The model under review builds one solid part; all positions refer to its coordinate system, in mm. Give positions to 0.01 mm unless a question says otherwise; leave off trailing zeros. Loops run counter-clockwise (first coordinate to the right, second up) from the corner with the lowest first, then second, coordinate; pieces in that order, holes last. Notation, with made-up numbers: (16, 27) - (20, 27) arc R23 ccw to (20, 59) - close; hole circle Ø9 at (53.5, 85). An arc over 180 degrees is marked (long way). Return JSON: item names as keys, results as strings. Group by question number.
```python
from build123d import *

# Parameters (mm, degrees)
SKETCH1_W                                 = 63.5
SKETCH1_H                                 = 19.05
BOSS_EXTRUDE1_DEPTH                       = 1.27
CSK_FOR_4_FLAT_HEAD_MACHINE_SCREW_2_COUNT = 2
CSK_FOR_4_FLAT_HEAD_MACHINE_SCREW_2_PITCH = 51.93240976
FILLET2_R                                 = 0.254


with BuildPart() as part:
    # Sketch1 → Boss-Extrude1 (new body)
    with BuildSketch(Plane(origin=(0, 0, 0), x_dir=(1, 0, 0), z_dir=(0, 1, 0))):
        with Locations((0, 21.324911643)):
            Rectangle(SKETCH1_W, SKETCH1_H)
    extrude(amount=BOSS_EXTRUDE1_DEPTH)

    # Sketch15 → CSK for #4 Flat Head Machine Screw (100)2 (revolve, cut)
    with BuildSketch(Plane(origin=(-25.96620488, 1.27, -21.930009473), x_dir=(0, 0, 1), z_dir=(1, 0, 0))):
        Polygon((0, 0), (0, 1.27), (1.63195, 1.27), (1.63195, 1.028358553), (2.8575, 0), align=None)
    csk_for_4_flat_head_machine_screw_100 = revolve(axis=Axis((-25.96620488, 7.62, -21.930009473), (0, -1, 0)), mode=Mode.SUBTRACT)

    # CSK for _4 Flat Head Machine Screw _ 2: CSK for #4 Flat Head Machine Screw (100)2 ×2
    with Locations(*[(i * CSK_FOR_4_FLAT_HEAD_MACHINE_SCREW_2_PITCH, 0, 0) for i in range(1, CSK_FOR_4_FLAT_HEAD_MACHINE_SCREW_2_COUNT)]):
        add(csk_for_4_flat_head_machine_screw_100, mode=Mode.SUBTRACT)

    # Fillet2
    fillet2_edges = [part.edges().sort_by_distance(p)[0] for p in [
        (-31.75, 1.27, -21.324911643),
        (0, 1.27, -11.799911643),
        (31.75, 1.27, -21.324911643),
        (0, 1.27, -30.849911643),
    ]]
    fillet(fillet2_edges, radius=FILLET2_R)


solid = part.part
```
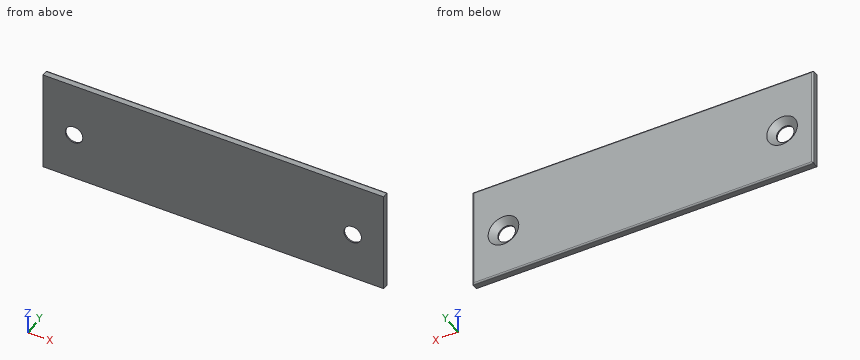
1) To check wall thickness, follow line 1 (X direction, y = 1.05, z = -19.75); line 2 (Z direction, x = -26, y = 0.1); line 3 (Z direction, x = -24, y = 0.85). State the ranges of each line that lie inside material, in increasing order.
2) For pin 1 Ø2 at (x, z) = (25.97, -21.93) entering from -Y; pin 2 Ø5 at (x, z) = (-25.97, -21.93) entering from +Y, all flat-tipped, find the tip position at first contact; note any pin that passes through.
3) We need section B-B, the plane z = -22.75. Count the separate pieces of the cut face and the enclosed holes in it, plus the area to 3 significant figures.
4) We need section A-A, the plane y = 0.75. Write out the cut boundary in (x, z), plus the area to 3 significant figures.
Findings:
{
 "1": {"line 1": "x = -31.75 to -27.37, -24.56 to 24.56, 27.37 to 31.75", "line 2": "z = -30.85 to -23.56, -20.3 to -11.8", "line 3": "z = -30.85 to -23.23, -20.63 to -11.8"},
 "2": {"pin 1": "passes through", "pin 2": "stops at y = 0.97"},
 "3": {"separate pieces": "3", "enclosed holes": "0", "area": "70.7 mm^2"},
 "4": {"outline": "(-31.75, -30.85) - (31.75, -30.85) - (31.75, -11.8) - (-31.75, -11.8) - close; hole circle Ø4.48 at (-25.97, -21.93); hole circle Ø4.48 at (25.97, -21.93)", "area": "1,180 mm^2"}
}
